from build123d import *

# Parameters (mm, degrees)
ESQUISSE1_W          = 50
ESQUISSE1_H          = 50
BOSS_EXTRU_1_DEPTH   = 2
ESQUISSE3_W          = 39.43
ESQUISSE3_H          = 1.87
BOSS_EXTRU_2_DEPTH   = 17.16
ESQUISSE4_W          = 39.43
ESQUISSE4_H          = 1.87
BOSS_EXTRU_3_DEPTH   = 5
D_GAGEMENT_M31_D     = 3.6
D_GAGEMENT_M31_DEPTH = 1.99
D_GAGEMENT_M31_TIP   = 1.081549114
ESQUISSE7_W          = 39.43
ESQUISSE7_H          = 1.87
BOSS_EXTRU_4_DEPTH   = 1.87


with BuildPart() as part:
    # Esquisse1 → Boss.-Extru.1 (new body)
    with BuildSketch(Plane(origin=(0, 0, 0), x_dir=(1, 0, 0), z_dir=(0, 1, 0))):
        with Locations((25, 25)):
            Rectangle(ESQUISSE1_W, ESQUISSE1_H)
    extrude(amount=BOSS_EXTRU_1_DEPTH)

    # Esquisse3 → Boss.-Extru.2 (add)
    with BuildSketch(Plane.XZ):
        with Locations((25, -49.065)):
            Rectangle(ESQUISSE3_W, ESQUISSE3_H)
        with Locations((25, -0.935)):
            Rectangle(ESQUISSE3_W, ESQUISSE3_H)
    extrude(amount=BOSS_EXTRU_2_DEPTH)

    # Esquisse4 → Boss.-Extru.3 (add)
    with BuildSketch(Plane(origin=(0, 0, -1.87), x_dir=(-1, 0, 0), z_dir=(0, 0, -1))):
        with Locations((-25, -16.225)):
            Rectangle(ESQUISSE4_W, ESQUISSE4_H)
    extrude(amount=BOSS_EXTRU_3_DEPTH)

    # Dégagement M31
    with Locations(Plane(origin=(36.195, -15.29, -4.37), x_dir=(0, 0, 1), z_dir=(0, 1, 0))):
        with Locations((0, 0), (0, -22.39)):
            Hole(D_GAGEMENT_M31_D / 2, depth=D_GAGEMENT_M31_DEPTH)
            with Locations((0, 0, -(D_GAGEMENT_M31_DEPTH + D_GAGEMENT_M31_TIP / 2))):  # 118° drill point
                Cone(0, D_GAGEMENT_M31_D / 2, D_GAGEMENT_M31_TIP, mode=Mode.SUBTRACT)

    # Esquisse7 → Boss.-Extru.4 (add)
    with BuildSketch(Plane.XZ.offset(17.16)):
        with Locations((25, -49.065)):
            Rectangle(ESQUISSE7_W, ESQUISSE7_H)
    extrude(amount=BOSS_EXTRU_4_DEPTH)


solid = part.part
Can you work these out from the model? Positions are in its coordinate system, mm. A direction names the side the tool comes from. Coordinates: 2 decimals unless noted, no trailing zeros. Order: outer loops, then holes, each group sorted by start corner. A loop starts at its lowest first (then second) coordinate and runs counter-clockwise, first axis right, second up. Notation, with made-up numbers: (2, 82.25) - (10, 82.25) arc R8 cw to (10, 95.25) - close; hole circle Ø7 at (43.5, -6.5). An arc over 180 degrees is marked (long way). Answer as a JSON object with one key per item and string values. Group by question number.
Q1. I need wall thicknesses on line 1 (Y direction, x = 12, z = -4); line 2 (Z direction, x = 24.5, y = -12); line 3 (Z direction, x = 43.5, y = -16.5). Which ranges of each line are inside material? Lowest first, please. Write a range as from..to.
Q2. Imagine slicing it at A-A (y = -3.25). Please give me the cut outline in (x, z) (3 decimals).
Q3. Will these pins go through, and if not, where does the flat tip stop? P1, Ø2, axis at y = -10.5, z = -49.5, coming from the +X side (3 decimals); P2, Ø1.5, axis at x = 5, z = -20, coming from the -Y side; P3, Ø5.5, axis at y = -10.5, z = -4, coming from the -X side (3 decimals); P4, Ø5, axis at y = -13.5, z = -10, coming from the +X side.
Q4. Imagine slicing it at B-B (z = -4.37). Please give me the cut outline in (x, y) (3 decimals), and give its area (3 significant figures).
Q5. On a 3-axis mill with a long thin cutter (end or side, diameter ignored), from which of +Z, -Z, +X, -X, +Y, -Y can I reach the whole of each face in a straight line? I mean faces 5 (the face through (25, -9, -48.13)), 6 (the face through (5.285, -11, -1)), 7 (the face through (44.715, -11, -1)), 8 (the face through (12.21, -16.24, -5.2)), 9 (the face through (25, -17.16, -3)). Say none if no direction works.
Q6. We'd pull the mould along Y, two halves only. Please class faces 1 (the face through (25, 2, -25)), 2 (the face through (25, -19.03, -49)), 3 (the face through (25, -8, -50)), 4 (the face through (25, -15.29, -4)): +Y half, -Y half, draft (parallel to the pull), parting line (faces both ways), or undercut.
Q7. Imagine slicing it at D-D (x = 14.5). Please give me the cut outline in (y, z).
Q8. Imagine slicing it at C-C (x = 24). Please give me the cut outline in (y, z), and give its area (3 significant figures).
Determined:
{
 "1": {"line 1": "y = -17.16..-15.29, 0..2", "line 2": "z = -50..-48.13, -1.87..0", "line 3": "z = -50..-48.13, -6.87..0"},
 "2": {"outline": "(5.285, -50) - (44.715, -50) - (44.715, -48.13) - (5.285, -48.13) - close; (5.285, -1.87) - (44.715, -1.87) - (44.715, 0) - (5.285, 0) - close"},
 "3": {"P1": "stops at x = 44.715", "P2": "stops at y = 0", "P3": "stops at x = 5.285", "P4": "passes through"},
 "4": {"outline": "(0, 0) - (50, 0) - (50, 2) - (0, 2) - close; (5.285, -17.16) - (12.005, -17.16) - (12.005, -15.29) - (5.285, -15.29) - close; (15.605, -17.16) - (34.395, -17.16) - (34.395, -15.29) - (15.605, -15.29) - close; (37.995, -17.16) - (44.715, -17.16) - (44.715, -15.29) - (37.995, -15.29) - close", "area": "160 mm2"},
 "5": {"face 5": "+X, -X, -Y", "face 6": "+Z, -Z, -X, -Y", "face 7": "+Z, -Z, +X, -Y", "face 8": "-Y", "face 9": "+Z, +X, -X, -Y"},
 "6": {"face 1": "+Y half", "face 2": "-Y half", "face 3": "draft", "face 4": "undercut"},
 "7": {"outline": "(-19.03, -50) - (2, -50) - (2, 0) - (-17.16, 0) - (-17.16, -2.71) - (-15.29, -2.71) - (-15.29, -1.87) - (0, -1.87) - (0, -48.13) - (-19.03, -48.13) - close; (-17.16, -6.87) - (-15.29, -6.87) - (-15.29, -6.03) - (-17.16, -6.03) - close"},
 "8": {"outline": "(-19.03, -50) - (2, -50) - (2, 0) - (-17.16, 0) - (-17.16, -6.87) - (-15.29, -6.87) - (-15.29, -1.87) - (0, -1.87) - (0, -48.13) - (-19.03, -48.13) - close", "area": "177 mm2"}
}
